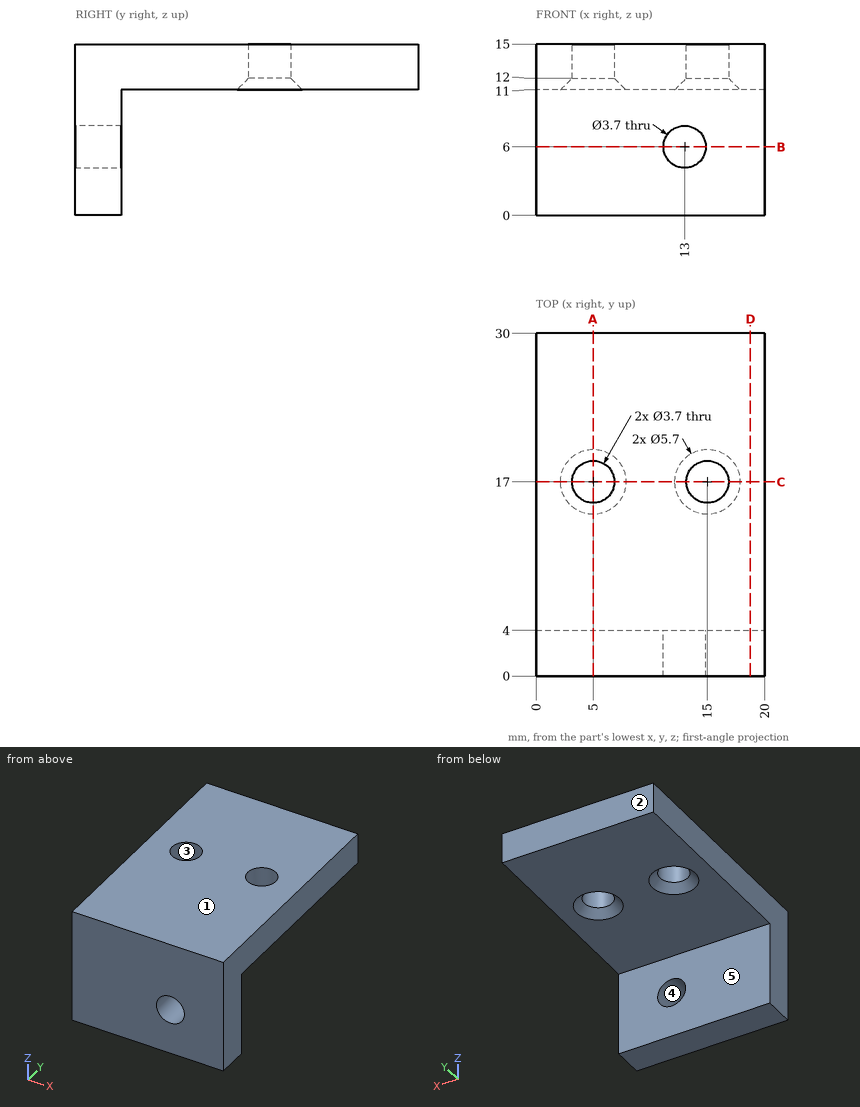
Answer from the drawing. Dimensions are ordinates in mm from the lowest x, y and z of the part. A direction names the side the tool comes from. Give positions to 0.01 mm unless a question says otherwise; leave off trailing zeros. Loops run counter-clockwise (first coordinate to the right, second up) from the corner with the lowest first, then second, coordinate; pieces in that order, holes last. Notation, with made-up numbers: (77, 13) - (99, 13) arc R11 cw to (99, 29) - close; hole circle Ø11 at (65, -2.5). An arc over 180 degrees is marked (long way). Write each question's results on one line, items separated by ' | '.
1. For a pull along Y with two mould halves and no side action, classify the marked faces 1, 2 and 3 as +Y half, -Y half, draft (parallel to the pull), parting line (faces both ways), or undercut.
Resolved:
face 1: draft | face 2: +Y half | face 3: undercut
2. Flat-ended cylindrical pins translate along their axes: P1, Ø12, axis at x = 12.5, y = 26.5, coming from the -Z side; P2, Ø4.5, axis at x = 13, z = 6, coming from the +Y side. Find the tip coordinate at first contact, or state that the pin passes through.
Resolved:
P1: stops at z = 11 | P2: stops at y = 4
3. Which of the six approach directions +Z, -Z, +X, -X, +Y, -Y give full straight-line access (tool end or side, diameter ignored) to the marked faces 4 and 5?
Resolved:
face 4: +Y, -Y | face 5: -Z, +X, -X, +Y
4. Find section D-D, the plane x = 18.75. Write down the section's boundary in (y, z).
Resolved:
outline: (0, 0) - (4, 0) - (4, 11) - (30, 11) - (30, 15) - (0, 15) - close
5. Find section C-C, the plane y = 17. Write down the section's boundary in (x, z), then the cut area to 3 significant figures.
Resolved:
outline: (0, 11) - (2.15, 11) - (3.15, 12) - (3.15, 15) - (0, 15) - close; (6.85, 12) - (7.85, 11) - (12.15, 11) - (13.15, 12) - (13.15, 15) - (6.85, 15) - close; (16.85, 12) - (17.85, 11) - (20, 11) - (20, 15) - (16.85, 15) - close | area: 48.4 mm^2
6. Find section B-B, the plane z = 6. Write down the section's boundary in (x, y).
Resolved:
outline: (0, 0) - (11.15, 0) - (11.15, 4) - (0, 4) - close; (14.85, 0) - (20, 0) - (20, 4) - (14.85, 4) - close
7. Consider probe 1 along Y at (x, z) = (15, 14.2); probe 2 along X at (y, z) = (1.4, 6); probe 3 along X at (y, z) = (18.5, 13). Determine where each line is inside the solid, lowest interval first. Write a range as from..to.
Resolved:
probe 1: y = 0..15.15, 18.85..30 | probe 2: x = 0..11.15, 14.85..20 | probe 3: x = 0..3.92, 6.08..13.92, 16.08..20
8. Find section A-A, the plane x = 5. Write down the section's boundary in (y, z).
Resolved:
outline: (0, 0) - (4, 0) - (4, 11) - (14.15, 11) - (15.15, 12) - (15.15, 15) - (0, 15) - close; (18.85, 12) - (19.85, 11) - (30, 11) - (30, 15) - (18.85, 15) - close
